```python
from build123d import *

# Parameters (mm, degrees)
F0_W     = 60
F0_H     = 44.8
F1_DEPTH = 9.9
F0_H_2   = 7.6
F2_DEPTH = 55.2
F3_START = 52.2
F0_H_3   = 10
F0_R     = 1.7
F3_DEPTH = 3
F4_START = 52.2
F4_DEPTH = 0.3
F5_START = 54.7
F5_DEPTH = 0.5


with BuildPart() as f1:
    # F0 (on Top) → F1 (new body)
    with BuildSketch(Plane.XY):
        Rectangle(F0_W, F0_H)
    extrude(amount=F1_DEPTH)

    # F0 (on Top) → F2 (join)
    with BuildSketch(Plane.XY):
        with Locations((0, -26.2)):
            Rectangle(F0_W, F0_H_2)
        with Locations((0, 26.2)):
            Rectangle(F0_W, F0_H_2)
    extrude(amount=F2_DEPTH)

    # F0 (on Top) → F3 (join)
    with BuildSketch(Plane.XY.offset(F3_START)):
        with Locations((0, 35)):
            Rectangle(F0_W, F0_H_3)
        with Locations((-15, 35)):
            Circle(F0_R, mode=Mode.SUBTRACT)
        with Locations((15, 35)):
            Circle(F0_R, mode=Mode.SUBTRACT)
        with Locations((0, -35)):
            Rectangle(F0_W, F0_H_3)
        with Locations((-15, -35)):
            Circle(F0_R, mode=Mode.SUBTRACT)
        with Locations((15, -35)):
            Circle(F0_R, mode=Mode.SUBTRACT)
    extrude(amount=F3_DEPTH)

    # F0 (on Top) → F4 (join)
    with BuildSketch(Plane.XY.offset(F4_START)):
        with Locations((-15, 35)):
            Circle(F0_R)
        with Locations((15, 35)):
            Circle(F0_R)
        with Locations((-15, -35)):
            Circle(F0_R)
        with Locations((15, -35)):
            Circle(F0_R)
    extrude(amount=F4_DEPTH)

    # F0 (on Top) → F5 (join)
    with BuildSketch(Plane.XY.offset(F5_START)):
        with Locations((-15, 35)):
            Circle(F0_R)
        with Locations((15, 35)):
            Circle(F0_R)
        with Locations((-15, -35)):
            Circle(F0_R)
        with Locations((15, -35)):
            Circle(F0_R)
    extrude(amount=F5_DEPTH)


solid = f1.part
```
Input: part model. Units: mm. Frame: model coordinates. A direction names the side the tool comes from. Coordinates: 2 decimals unless noted, no trailing zeros. Order: outer loops, then holes, each group sorted by start corner. A loop starts at its lowest first (then second) coordinate and runs counter-clockwise, first axis right, second up. Notation, with made-up numbers: (-32, 63) - (-16, 63) arc R25 ccw to (-16, 89) - close; hole circle Ø4 at (60, -21.5). An arc over 180 degrees is marked (long way). Return JSON: item names as keys, results as strings.
Q1. Cut plane B-B (x = 23.5). Return loops of the section in (y, z).
The answers:
{"outline": "(-40, 52.2) - (-30, 52.2) - (-30, 0) - (30, 0) - (30, 52.2) - (40, 52.2) - (40, 55.2) - (22.4, 55.2) - (22.4, 9.9) - (-22.4, 9.9) - (-22.4, 55.2) - (-40, 55.2) - close"}
Q2. Access query for faces 5 (the flat face through (0, -30, 26)), 6 (the flat face through (-30, 0, 9)), 7 (the flat face through (-15, -35, 52.5)), 8 (the flat face through (0, -40, 54)), 9 (the flat face through (0, 22.4, 32)). Directions: +Z, -Z, +X, -X, +Y, -Y. A direction counts if a zero-diameter tool reaches every point of the face in a straight line with its end or side. Return the directions, or none.
The answers:
{"face 5": "-Z, +X, -X, -Y", "face 6": "+Z, -Z, -X, +Y, -Y", "face 7": "none", "face 8": "+Z, -Z, +X, -X, -Y", "face 9": "+Z, +X, -X"}
Q3. Cut plane A-A (z = 47.5). Return loops of the section in (x, y), then the cut area to 3 significant figures.
The answers:
{"outline": "(-30, -30) - (30, -30) - (30, -22.4) - (-30, -22.4) - close; (-30, 22.4) - (30, 22.4) - (30, 30) - (-30, 30) - close", "area": "912 mm2"}
Q4. Ray query, probe 1 along Y at (x, z) = (15, 53); probe 2 along Y at (x, z) = (18.5, 47.5); probe 3 along Z at (x, y) = (5, 36.5). Return the intervals inside material, ascending.
The answers:
{"probe 1": "y = -40 to -36.7, -33.3 to -22.4, 22.4 to 33.3, 36.7 to 40", "probe 2": "y = -30 to -22.4, 22.4 to 30", "probe 3": "z = 52.2 to 55.2"}
Q5. Cut plane D-D (x = 15). Return loops of the section in (y, z), then the cut area to 3 significant figures.
The answers:
{"outline": "(-40, 52.2) - (-30, 52.2) - (-30, 0) - (30, 0) - (30, 52.2) - (40, 52.2) - (40, 55.2) - (22.4, 55.2) - (22.4, 9.9) - (-22.4, 9.9) - (-22.4, 55.2) - (-40, 55.2) - close; hole (-36.7, 52.5) - (-33.3, 52.5) - (-33.3, 54.7) - (-36.7, 54.7) - close; hole (33.3, 52.5) - (36.7, 52.5) - (36.7, 54.7) - (33.3, 54.7) - close", "area": "1,330 mm2"}
Q6. First-contact query: pin 1 (1.5 mm diameter, centred on x = -6, y = -13.5, fed in from +Z); pin 2 (2.5 mm diameter, centred on x = -15, y = 35.5, fed in from -Z); pin 3 (8 mm diameter, centred on x = -21, z = 36.5, fed in from +Y). Flat tips, straight axial feed; report the tip coordinate or a pass-through.
The answers:
{"pin 1": "stops at z = 9.9", "pin 2": "stops at z = 52.2", "pin 3": "stops at y = 30"}
Q7. Draft query along Z for faces 1 (the flat face through (0, 31, 55.2)), 2 (the flat face through (0, -35, 52.2)), 3 (the cylindrical face through (15.8, 33.5, 53.6)), 4 (the flat face through (0, -22.4, 32)). Return one class per face: +Z half, -Z half, draft (parallel to the pull), parting line (faces both ways), or undercut.
The answers:
{"face 1": "+Z half", "face 2": "-Z half", "face 3": "undercut", "face 4": "draft"}
Q8. Cut plane C-C (y = -35). Return loops of the section in (x, z).
The answers:
{"outline": "(-30, 52.2) - (30, 52.2) - (30, 55.2) - (-30, 55.2) - close; hole (-16.7, 52.5) - (-13.3, 52.5) - (-13.3, 54.7) - (-16.7, 54.7) - close; hole (13.3, 52.5) - (16.7, 52.5) - (16.7, 54.7) - (13.3, 54.7) - close"}
